Geometry check sheet. Reference: the model listing, model coordinates, mm. A direction names the side the tool comes from. Coordinates: 2 decimals unless noted, no trailing zeros. Loops run counter-clockwise (first coordinate to the right, second up) from the corner with the lowest first, then second, coordinate; pieces in that order, holes last.
from build123d import *

# Parameters (mm, degrees)
SKETCH1_R           = 15
BOSS_EXTRUDE1_DEPTH = 50
SKETCH2_R           = 5
CUT_EXTRUDE1_DEPTH  = 20
SKETCH3_R           = 5
CUT_EXTRUDE2_DEPTH  = 10


with BuildPart() as part:
    # Sketch1 → Boss-Extrude1 (new body)
    with BuildSketch(Plane(origin=(0, 0, 0), x_dir=(1, 0, 0), z_dir=(0, 1, 0))):
        Circle(SKETCH1_R)
    extrude(amount=BOSS_EXTRUDE1_DEPTH)

    # Sketch2 → Cut-Extrude1 (cut)
    with BuildSketch(Plane.ZY.offset(25)):
        with Locations((0, 25)):
            Circle(SKETCH2_R)
    extrude(amount=-CUT_EXTRUDE1_DEPTH, mode=Mode.SUBTRACT)

    # Sketch3 → Cut-Extrude2 (cut)
    with BuildSketch(Plane(origin=(0, 50, 0), x_dir=(1, 0, 0), z_dir=(0, 1, 0))):
        Circle(SKETCH3_R)
    extrude(amount=-CUT_EXTRUDE2_DEPTH, mode=Mode.SUBTRACT)


solid = part.part
1) Access from +Z, -Z, +X, -X, +Y, -Y to the whole of each face (thin tool, end or side, straight path). Record for faces 4 (the cylindrical face through (-1.08, 45.07, 4.88)), 5 (the cylindrical face through (-10.073, 29.957, -0.651)), 6 (the flat face through (-4, 50, -4)).
Data:
face 4: +Y
face 5: -X
face 6: +Z, -Z, +X, -X, +Y
2) Section check D-D on y = 7. Record the cut outline in (x, z).
Data:
outline: circle Ø30 at (0, 0)
3) Material ranges on probe 1 along Z at (x, y) = (0, 45.5); probe 2 along X at (y, z) = (18, 0.5), recorded low to high.
Data:
probe 1: z = -15 to -5, 5 to 15
probe 2: x = -14.99 to 14.99
4) Section check C-C on z = 0. Record the cut outline in (x, y), and give its area (3 significant figures).
Data:
outline: (-15, 0) - (15, 0) - (15, 50) - (5, 50) - (5, 40) - (-5, 40) - (-5, 50) - (-15, 50) - (-15, 30) - (-5, 30) - (-5, 20) - (-15, 20) - close
area: 1,300 mm2
5) Depth check by flat-ended pin: pin 1 (5 mm diameter, centred on x = -6.5, z = -9, fed in from -Y); pin 2 (8 mm diameter, centred on y = 22.5, z = 11.5, fed in from +X); pin 3 (1 mm diameter, centred on y = 39.5, z = 12, fed in from +X); pin 4 (5 mm diameter, centred on x = -3.5, y = 13, fed in from -Z). Enter the tip coordinate at first touch or a pass-through.
Data:
pin 1: stops at y = 0
pin 2: stops at x = 12.99
pin 3: stops at x = 9.63
pin 4: stops at z = -14.97
6) Section check B-B on y = 44. Record the cut outline in (x, z), and give its area (3 significant figures).
Data:
outline: circle Ø30 at (0, 0); hole circle Ø10 at (0, 0)
area: 628 mm2
7) Section check A-A on x = 0. Record the cut outline in (y, z), and give its area (3 significant figures).
Data:
outline: (0, -15) - (50, -15) - (50, -5) - (40, -5) - (40, 5) - (50, 5) - (50, 15) - (0, 15) - close
area: 1,400 mm2
8) Mould release check, pull along Z, two halves, no side actions. Record for faces 1 (the cylindrical face through (13.856, 24.65, 5.745)), 2 (the flat face through (0, 40, 0)), 3 (the flat face through (0, 0, 0)): +Z half, -Z half, draft (parallel to the pull), parting line (faces both ways), or undercut.
Data:
face 1: parting line
face 2: undercut
face 3: draft
